Work out the finished part from the listing and answer in its coordinate system (mm). A direction names the side the tool comes from. Round coordinates to 2 decimals unless told otherwise and drop trailing zeros. Order: outer loops, then holes, each group sorted by start corner. A loop starts at its lowest first (then second) coordinate and runs counter-clockwise, first axis right, second up. Notation, with made-up numbers: (71, 1) - (118, 1) arc R30 ccw to (118, 27) - close; hole circle Ø9 at (81, -38). An arc over 180 degrees is marked (long way). Put each result on its own line as item: value.
```python
from build123d import *

# Parameters (mm, degrees)
SKETCH_6_W      = 120
SKETCH_6_H      = 113.017251625
SKETCH_6_R      = 1.75
EXTRUDE_2_DEPTH = 3.6
FILLET_1_R      = 30
FILLET_2_R      = 30


with BuildPart() as part:
    # 草图6 → 凸台-拉伸2 (new body)
    with BuildSketch(Plane(origin=(0, 0, 0), x_dir=(1, 0, 0), z_dir=(0, 1, 0))):
        with Locations((95, 83.491374187)):
            Rectangle(SKETCH_6_W, SKETCH_6_H)
        with Locations((43.263065037, 32.093294966)):
            Circle(SKETCH_6_R, mode=Mode.SUBTRACT)
        with Locations((67.163065037, 32.093294966)):
            Circle(SKETCH_6_R, mode=Mode.SUBTRACT)
        with BuildLine():
            ThreePointArc((79.1225441, 38.232748375), (77.3725441, 39.982748375), (79.1225441, 41.732748375))
            Line((79.1225441, 41.732748375), (110.8774559, 41.732748375))
            ThreePointArc((110.8774559, 41.732748375), (112.6274559, 39.982748375), (110.8774559, 38.232748375))
            Line((110.8774559, 38.232748375), (79.1225441, 38.232748375))
        make_face(mode=Mode.SUBTRACT)
        with Locations((43.263065037, 62.193294966)):
            Circle(SKETCH_6_R, mode=Mode.SUBTRACT)
        with Locations((67.163065037, 62.193294966)):
            Circle(SKETCH_6_R, mode=Mode.SUBTRACT)
        with Locations((75.95, 132)):
            Circle(SKETCH_6_R, mode=Mode.SUBTRACT)
        with Locations((114.05, 132)):
            Circle(SKETCH_6_R, mode=Mode.SUBTRACT)
        with Locations((122.836934963, 62.193294966)):
            Circle(SKETCH_6_R, mode=Mode.SUBTRACT)
        with Locations((122.836934963, 32.093294966)):
            Circle(SKETCH_6_R, mode=Mode.SUBTRACT)
        with Locations((146.736934963, 32.093294966)):
            Circle(SKETCH_6_R, mode=Mode.SUBTRACT)
        with Locations((146.736934963, 62.193294966)):
            Circle(SKETCH_6_R, mode=Mode.SUBTRACT)
    extrude(amount=EXTRUDE_2_DEPTH)

    # 圆角1
    fillet_1_edges = [part.edges().sort_by_distance(p)[0] for p in [
        (35, 1.8, -140),
    ]]
    fillet(fillet_1_edges, radius=FILLET_1_R)

    # 圆角2
    fillet_2_edges = [part.edges().sort_by_distance(p)[0] for p in [
        (155, 1.8, -140),
    ]]
    fillet(fillet_2_edges, radius=FILLET_2_R)


solid = part.part
```
1) Given pin 1 Ø2 at (x, z) = (82.5, -124) entering from -Y, flat-ended and moving along its own axis, determine where the tip first touches the part or whether it passes through.
Findings below:
pin 1: stops at y = 0
2) A cutting plane is placed at C-C on y = 1.55. Give the number of separate pieces and of enclosed holes in the cut face, then the cut area to 3 significant figures.
Findings below:
separate pieces: 1
enclosed holes: 11
area: 13,000 mm2
3) A cutting plane is placed at B-B on z = -132. Write down the section's boundary in (x, y), then the cut area to 3 significant figures.
Findings below:
outline: (44.6, 0) - (74.2, 0) - (74.2, 3.6) - (44.6, 3.6) - close; (77.7, 0) - (112.3, 0) - (112.3, 3.6) - (77.7, 3.6) - close; (115.8, 0) - (145.4, 0) - (145.4, 3.6) - (115.8, 3.6) - close
area: 338 mm2
4) For a pull along Z with two mould halves and no side action, classify faces 1 (the flat face through (94, 0, -84)), 2 (the flat face through (95, 2, -140)), 3 (the flat face through (94, 2, -26.983)), 4 (the flat face through (95, 2, -41.733)) as pulls with the +Z half, pulls with the -Z half, needs draft (parallel to the pull), parting line crosses it, or undercut.
Findings below:
face 1: needs draft
face 2: pulls with the -Z half
face 3: pulls with the +Z half
face 4: undercut
5) Straight lines are drawn through the part: L1, parallel to Z at x = 121.5, y = 1.3; L2, parallel to Z at x = 123.5, y = 2.65; L3, parallel to Z at x = 104, y = 0.2. For each, find the intervals that lie inside material, in ascending order. Write a range as from..to.
Findings below:
L1: z = -140..-63.32, -61.06..-33.22, -30.96..-26.98
L2: z = -140..-63.81, -60.57..-33.71, -30.47..-26.98
L3: z = -140..-41.73, -38.23..-26.98
6) For faces 5 (the cylindrical face through (43.555, 1.825, -130.979)), 6 (the cylindrical face through (77.373, 1.775, -39.944)), determine the directions among +Z, -Z, +X, -X, +Y, -Y from which every point of the face is accessible in a straight line to the end or side of a thin tool.
Findings below:
face 5: -Z, -X, +Y, -Y
face 6: +Y, -Y
7) A cutting plane is placed at A-A on x = 114.05. Write down the section's boundary in (y, z).
Findings below:
outline: (0, -140) - (3.6, -140) - (3.6, -133.75) - (0, -133.75) - close; (0, -130.25) - (3.6, -130.25) - (3.6, -26.98) - (0, -26.98) - close
